```python
from build123d import *

# Parameters (mm, degrees)
SKETCH_1_W          = 61
SKETCH_1_H          = 46
EXTRUDE_1_DEPTH     = 31
CUT_EXTRUDE_1_DEPTH = 28.5
SKETCH_3_R          = 2.5
CUT_EXTRUDE_2_DEPTH = 28.5
CUT_EXTRUDE_3_DEPTH = 28.5
CUT_EXTRUDE_4_DEPTH = 68.5
CUT_EXTRUDE_5_DEPTH = 2
CUT_EXTRUDE_6_DEPTH = 2
SKETCH_8_R          = 3
CUT_EXTRUDE_7_DEPTH = 7.2
CUT_EXTRUDE_8_DEPTH = 10
CUT_EXTRUDE_9_DEPTH = 10
FILLET_1_R          = 3


with BuildPart() as part:
    # 草图1 → 凸台-拉伸1 (new body)
    with BuildSketch(Plane.XY):
        with Locations((30.5, 23)):
            Rectangle(SKETCH_1_W, SKETCH_1_H)
    extrude(amount=EXTRUDE_1_DEPTH)

    # 草图2 → 切除-拉伸1 (cut)
    with BuildSketch(Plane.XY.offset(31)):
        with BuildLine():
            ThreePointArc((7, 18), (10.535533906, 19.464466094), (12, 23))
            ThreePointArc((12, 23), (10.535533906, 26.535533906), (7, 28))
            Line((7, 28), (0, 28))
            Line((0, 28), (0, 18))
            Line((0, 18), (7, 18))
        make_face()
        with BuildLine():
            Line((61, 18), (61, 28))
            Line((61, 28), (54, 28))
            ThreePointArc((54, 28), (49, 23), (54, 18))
            Line((54, 18), (61, 18))
        make_face()
    extrude(amount=-CUT_EXTRUDE_1_DEPTH, mode=Mode.SUBTRACT)

    # 草图3 → 切除-拉伸2 (cut)
    with BuildSketch(Plane.XY.offset(2.5)):
        with Locations((5.7, 23)):
            Circle(SKETCH_3_R)
    extrude(amount=-CUT_EXTRUDE_2_DEPTH, mode=Mode.SUBTRACT)

    # 草图4 → 切除-拉伸3 (cut)
    with BuildSketch(Plane.XY.offset(2.5)):
        with BuildLine():
            Line((53.3, 25.5), (55.3, 25.5))
            ThreePointArc((55.3, 25.5), (57.8, 23), (55.3, 20.5))
            Line((55.3, 20.5), (53.3, 20.5))
            ThreePointArc((53.3, 20.5), (50.8, 23), (53.3, 25.5))
        make_face()
    extrude(amount=-CUT_EXTRUDE_3_DEPTH, mode=Mode.SUBTRACT)

    # 草图5 → 切除-拉伸4 (cut)
    with BuildSketch(Plane.XZ):
        Polygon((30.5, 31), (46.85, 31), (46.85, 29), (14.15, 29), (14.15, 31), align=None)
    extrude(amount=-CUT_EXTRUDE_4_DEPTH, mode=Mode.SUBTRACT)

    # 草图6 → 切除-拉伸5 (cut)
    with BuildSketch(Plane.XZ):
        with BuildLine():
            Line((14.15, 29), (46.85, 29))
            ThreePointArc((46.85, 29), (30.5, 27.654333407), (14.15, 29))
        make_face()
    extrude(amount=-CUT_EXTRUDE_5_DEPTH, mode=Mode.SUBTRACT)

    # 草图7 → 切除-拉伸6 (cut)
    with BuildSketch(Plane(origin=(0, 46, 0), x_dir=(1, 0, 0), z_dir=(0, 1, 0))):
        with BuildLine():
            Line((14.15, -29), (46.85, -29))
            ThreePointArc((46.85, -29), (30.5, -27.654333407), (14.15, -29))
        make_face()
    extrude(amount=-CUT_EXTRUDE_6_DEPTH, mode=Mode.SUBTRACT)

    # 草图8 → 切除-拉伸7 (cut)
    with BuildSketch(Plane.XY.offset(31)):
        with BuildLine():
            ThreePointArc((10, 37), (9.121320344, 39.121320344), (7, 40))
            Line((7, 40), (7, 37))
            Line((7, 37), (4, 37))
            ThreePointArc((4, 37), (7, 34), (10, 37))
        make_face()
        with BuildLine():
            Line((7, 37), (7, 40))
            ThreePointArc((7, 40), (4.878679656, 39.121320344), (4, 37))
            Line((4, 37), (7, 37))
        make_face()
        with Locations((7, 9)):
            Circle(SKETCH_8_R)
        with Locations((54, 9)):
            Circle(SKETCH_8_R)
        with Locations((54, 37)):
            Circle(SKETCH_8_R)
    extrude(amount=-CUT_EXTRUDE_7_DEPTH, mode=Mode.SUBTRACT)

    # 草图9 → 切除-拉伸8 (cut)
    with BuildSketch(Plane.ZY):
        Polygon((23.8, 32), (23.8, 37), (23.8, 42), (17.8, 42), (17.8, 41.5), (17.8, 32), align=None)
        Polygon((23.8, 4), (23.8, 14), (17.8, 14), (17.8, 4.5), (17.8, 4), align=None)
    extrude(amount=-CUT_EXTRUDE_8_DEPTH, mode=Mode.SUBTRACT)

    # 草图10 → 切除-拉伸9 (cut)
    with BuildSketch(Plane(origin=(61, 0, 0), x_dir=(0, 0, -1), z_dir=(1, 0, 0))):
        Polygon((-23.8, 4), (-23.8, 9), (-23.8, 14), (-17.8, 14), (-17.8, 4), align=None)
        Polygon((-23.8, 42), (-17.8, 42), (-17.8, 32), (-23.8, 32), (-23.8, 37), align=None)
    extrude(amount=-CUT_EXTRUDE_9_DEPTH, mode=Mode.SUBTRACT)

    # 圆角1
    fillet_1_edges = [part.edges().sort_by_distance(p)[0] for p in [
        (61, 9, 31),
        (0, 9, 31),
        (61, 37, 31),
        (0, 37, 31),
    ]]
    fillet(fillet_1_edges, radius=FILLET_1_R)


solid = part.part
```
For this review, take the finished solid that the model builds, in its own axes (mm). A direction names the side the tool comes from. Coordinates: 2 decimals unless noted, no trailing zeros. Write each loop counter-clockwise with the first axis right and the second up, starting at its lowest first coordinate (ties: lowest second). Pieces come first, ordered by that corner, then holes.
(1) For pin 1 Ø10 at (x, y) = (23, 20) entering from +Z; pin 2 Ø3 at (y, z) = (9.5, 20) entering from -X; pin 3 Ø3.5 at (x, y) = (7, 9) entering from +Z, all flat-tipped, find the tip position at first contact; note any pin that passes through.
(2) Add section A-A on z = 9. Give the boundary of the cut face in (x, y).
(3) Wall thickness on probe 1 along Y at (x, z) = (7, 27); probe 2 along X at (y, z) = (37, 27); probe 3 along Y at (x, z) = (5.7, 0.9): over which ranges is each line inside the solid? List them lowest first.
(4) The part is to be moulded in two halves that separate along X. For faces 6 (the face through (46.85, 23, 30)), 7 (the face through (0.86, 9.13, 30.1)), 8 (the face through (54, 25.5, 1)), 9 (the face through (30, 23, 0)), say which applies: +X half, -X half, draft (parallel to the pull), parting line (faces both ways), or undercut.
(5) Add section B-B on y = 38. Give the boundary of the cut face in (x, z), then the cut area to 3 significant figures.
(6) Add section D-D on z = 23. Give the boundary of the cut face in (x, y), then the cut area to 3 significant figures.
(7) Add section C-C on x = 28. Give the boundary of the cut face in (y, z).
(8) Tool access review of faces 1 (the face through (3, 18, 17)), 2 (the face through (30.73, 0.986, 27.655)), 3 (the face through (5, 14, 21)), 4 (the face through (9.77, 7.85, 27.45)), 5 (the face through (56, 42, 21)): name each direction out of +Z, -Z, +X, -X, +Y, -Y from which nothing blocks a thin tool from reaching the whole face with its end or side.
Answer sheet:
1. pin 1: stops at z = 29
1. pin 2: stops at x = 10
1. pin 3: stops at z = 17.8
2. outline: (0, 0) - (61, 0) - (61, 18) - (54, 18) arc R5 cw to (54, 28) - (61, 28) - (61, 46) - (0, 46) - (0, 28) - (7, 28) arc R5 cw to (7, 18) - (0, 18) - close
3. probe 1: y = 0 to 6, 12 to 18, 28 to 34, 40 to 46
3. probe 2: x = 0 to 4, 10 to 51, 57 to 61
3. probe 3: y = 0 to 20.5, 25.5 to 46
4. face 6: undercut
4. face 7: -X half
4. face 8: undercut
4. face 9: draft
5. outline: (0, 0) - (61, 0) - (61, 17.8) - (51, 17.8) - (51, 23.8) - (51.17, 23.8) - (51.17, 31) - (46.85, 31) - (46.85, 29) - (14.15, 29) - (14.15, 31) - (9.83, 31) - (9.83, 23.8) - (10, 23.8) - (10, 17.8) - (0, 17.8) - close; (0, 23.8) - (4.17, 23.8) - (4.17, 31) - (3, 31) arc R3 ccw to (0, 28) - close; (56.83, 23.8) - (61, 23.8) - (61, 28) arc R3 ccw to (58, 31) - (56.83, 31) - close
5. area: 1,620 mm2
6. outline: (0, 0) - (61, 0) - (61, 4) - (51, 4) - (51, 14) - (61, 14) - (61, 18) - (54, 18) arc R5 cw to (54, 28) - (61, 28) - (61, 32) - (51, 32) - (51, 42) - (61, 42) - (61, 46) - (0, 46) - (0, 42) - (10, 42) - (10, 32) - (0, 32) - (0, 28) - (7, 28) arc R5 cw to (7, 18) - (0, 18) - (0, 14) - (10, 14) - (10, 4) - (0, 4) - close
6. area: 2,190 mm2
7. outline: (0, 0) - (46, 0) - (46, 27.69) - (44, 27.69) - (44, 29) - (2, 29) - (2, 27.69) - (0, 27.69) - close
8. face 1: +Z, -X
8. face 2: +Z, -Y
8. face 3: -X
8. face 4: +Z
8. face 5: +X
